CAD build for the part. Positions are in the model's coordinates, mm. Round coordinates to 2 decimals unless told otherwise and drop trailing zeros. Loops run counter-clockwise (first coordinate to the right, second up) from the corner with the lowest first, then second, coordinate; pieces in that order, holes last. Notation, with made-up numbers: M -20,36 L 5,36 A22 cw 5,57 Z; hole C 83,47.5 d8. An arc over 180 degrees is marked long. One line per item, written item: value. Start each with the question number.
from build123d import *

# Parameters (mm, degrees)
F0_R     = 1.5
F0_R_2   = 1.8288
F0_R_3   = 11.253
F1_DEPTH = 1.70942
F2_R     = 3.96875


with BuildPart() as f1:
    # F0 (on Top) → F1 (new body)
    with BuildSketch(Plane.XY):
        with BuildLine():
            Line((-21.502992, 15.499982), (-21.502992, -15.499982))
            Line((-21.502992, -15.499982), (-15.499982, -21.502992))
            Line((-15.499982, -21.502992), (-4.105352, -28.812279))
            ThreePointArc((-4.105352, -28.812279), (-3.079023, -29.280202), (-1.962506, -29.440492))
            Line((-1.962506, -29.440492), (22.643744, -29.440492))
            Line((22.643744, -29.440492), (22.643744, 29.440492))
            Line((22.643744, 29.440492), (-1.962506, 29.440492))
            ThreePointArc((-1.962506, 29.440492), (-3.079023, 29.280202), (-4.105352, 28.812279))
            Line((-4.105352, 28.812279), (-15.499982, 21.502992))
            Line((-15.499982, 21.502992), (-21.502992, 15.499982))
        make_face()
        with Locations((-15.499994, -15.499994)):
            Circle(F0_R, mode=Mode.SUBTRACT)
        with Locations((-1.962506, -25.471742)):
            Circle(F0_R_2, mode=Mode.SUBTRACT)
        with Locations((18.674994, -25.471742)):
            Circle(F0_R_2, mode=Mode.SUBTRACT)
        with Locations((15.499994, -15.499994)):
            Circle(F0_R, mode=Mode.SUBTRACT)
        Circle(F0_R_3, mode=Mode.SUBTRACT)
        with Locations((-15.499994, 15.499994)):
            Circle(F0_R, mode=Mode.SUBTRACT)
        with Locations((-1.962506, 25.471742)):
            Circle(F0_R_2, mode=Mode.SUBTRACT)
        with Locations((15.499994, 15.499994)):
            Circle(F0_R, mode=Mode.SUBTRACT)
        with Locations((18.674994, 25.471742)):
            Circle(F0_R_2, mode=Mode.SUBTRACT)
    extrude(amount=F1_DEPTH)

    # F2
    f2_edges = [f1.edges().sort_by_distance(p)[0] for p in [
        (22.643744, -29.440492, 0.85471),
        (22.643744, 29.440492, 0.85471),
    ]]
    fillet(f2_edges, radius=F2_R)


solid = f1.part
(1) Flat gauge pin, fed straight in: P1, Ø2.5, axis at x = -15.5, y = -15.5, coming from the -Z side. Where does the tip first touch, or does it go through?
(2) Slice it at C-C, the plane x = 18. List the corners of the cut face in (y, z), and give its area (3 significant figures).
(3) Probe L1, parallel to Y at x = -15.5, z = 1.25; L2, parallel to X at y = 14.5, z = 0.2; L3, parallel to Y at x = -15, z = 1.1. List the from-to ranges inside material, lowest first.
(4) Slice it at A-A, the plane y = 0. List the corners of the cut face in (x, z).
(5) Slice it at D-D, the plane x = -10.5. List the corners of the cut face in (y, z).
(6) Slice it at B-B, the plane z = 1.25. Count the separate pieces of the cut face and the enclosed holes in it, and give its area (3 significant figures).
(7) Mould opens along Y. For faces 1 (the cylindrical face through (-3.064, 29.285, 0.843)), 2 (the cylindrical face through (20.364, -26.172, 0.843)), 3 (the flat face through (10, 7, 1.709)), 4 (the flat face through (-9.88, -25.11, 0.84)) say: pulls with the +Y half, pulls with the -Y half, needs draft (parallel to the pull), parting line crosses it, or undercut.
Check result:
1. P1: passes through
2. outline: M -29.44,0 L -27.17,0 L -27.17,1.71 L -29.44,1.71 Z; M -23.77,0 L 23.77,0 L 23.77,1.71 L -23.77,1.71 Z; M 27.17,0 L 29.44,0 L 29.44,1.71 L 27.17,1.71 Z
2. area: 89.0 mm^2
3. L1: y = -21.5 to -17, -14 to 14, 17 to 21.5
3. L2: x = -21.5 to -16.62, -14.38 to 14.38, 16.62 to 22.64
3. L3: y = -21.82 to -16.91, -14.09 to 14.09, 16.91 to 21.82
4. outline: M -21.5,0 L -11.25,0 L -11.25,1.71 L -21.5,1.71 Z; M 11.25,0 L 22.64,0 L 22.64,1.71 L 11.25,1.71 Z
5. outline: M -24.71,0 L -4.05,0 L -4.05,1.71 L -24.71,1.71 Z; M 4.05,0 L 24.71,0 L 24.71,1.71 L 4.05,1.71 Z
6. separate pieces: 1
6. enclosed holes: 9
6. area: 1,890 mm^2
7. face 1: pulls with the +Y half
7. face 2: undercut
7. face 3: needs draft
7. face 4: pulls with the -Y half
